```python
from build123d import *

# Parameters (mm, degrees)
SKETCH1_R           = 1.27
BOSS_EXTRUDE1_DEPTH = 2.5
FILLET1_R           = 5.08
CUT_EXTRUDE1_DEPTH  = 14.648809639
FILLET2_R           = 1.27


with BuildPart() as part:
    # Sketch1 → Boss-Extrude1 (new, symmetric)
    with BuildSketch(Plane(origin=(0, 0, 0), x_dir=(1, 0, 0), z_dir=(0, 1, 0))):
        with BuildLine():
            ThreePointArc((7.094482759, 2.780775861), (0, 7.62), (-7.094482759, 2.780775861))
            ThreePointArc((-7.094482759, 2.780775861), (-10.16, 0), (-7.094482759, -2.780775861))
            ThreePointArc((-7.094482759, -2.780775861), (0, -7.62), (7.094482759, -2.780775861))
            ThreePointArc((7.094482759, -2.780775861), (10.16, 0), (7.094482759, 2.780775861))
        make_face()
        with Locations(Location((7.366, 0, 0), (0, 0, 270))):
            Circle(SKETCH1_R, mode=Mode.SUBTRACT)
        with Locations(Location((-7.366, 0, 0), (0, 0, 270))):
            Circle(SKETCH1_R, mode=Mode.SUBTRACT)
    extrude(amount=BOSS_EXTRUDE1_DEPTH, both=True)

    # Fillet1
    fillet1_edges = [part.edges().sort_by_distance(p)[0] for p in [
        (-7.094482759, 0, 2.780775861),
        (-7.094482759, 0, -2.780775861),
        (7.094482759, 0, -2.780775861),
        (7.094482759, 0, 2.780775861),
    ]]
    fillet(fillet1_edges, radius=FILLET1_R)

    # Sketch2 → Cut-Extrude1 (cut, through all)
    with BuildSketch(Plane(origin=(0, 2.5, 0), x_dir=(1, 0, 0), z_dir=(0, 1, 0))):
        with BuildLine():
            ThreePointArc((5.213513626, 2.46164628), (4.096, 0), (5.213513626, -2.46164628))
            ThreePointArc((5.213513626, -2.46164628), (4.900166041, -2.826173582), (4.612275862, -3.21112307))
            ThreePointArc((4.612275862, -3.21112307), (0, -5.62), (-4.612275862, -3.21112307))
            ThreePointArc((-4.612275862, -3.21112307), (-4.900166041, -2.826173582), (-5.213513626, -2.46164628))
            ThreePointArc((-5.213513626, -2.46164628), (-4.096, 0), (-5.213513626, 2.46164628))
            ThreePointArc((-5.213513626, 2.46164628), (-4.900166041, 2.826173582), (-4.612275862, 3.21112307))
            ThreePointArc((-4.612275862, 3.21112307), (0, 5.62), (4.612275862, 3.21112307))
            ThreePointArc((4.612275862, 3.21112307), (4.900166041, 2.826173582), (5.213513626, 2.46164628))
        make_face()
    extrude(amount=-CUT_EXTRUDE1_DEPTH, mode=Mode.SUBTRACT)

    # Fillet2
    fillet2_edges = [part.edges().sort_by_distance(p)[0] for p in [
        (5.213513626, 0, -2.46164628),
        (-5.213513626, 0, -2.46164628),
        (-5.213513626, 0, 2.46164628),
        (5.213513626, 0, 2.46164628),
    ]]
    fillet(fillet2_edges, radius=FILLET2_R)


solid = part.part
```
The listing builds one solid part. Answer for the finished solid, in the listing's coordinates (mm). A direction names the side the tool comes from. Round coordinates to 2 decimals unless told otherwise and drop trailing zeros. Write each loop counter-clockwise with the first axis right and the second up, starting at its lowest first coordinate (ties: lowest second). Pieces come first, ordered by that corner, then holes. Notation, with made-up numbers: (-24, 14.25) -> (-18, 14.25) arc R18 ccw to (-18, 48.25) -> close; hole circle Ø6 at (-7.75, 85.25). An arc over 180 degrees is marked (long way). Answer as a JSON object with one key per item and string values. Group by question number.
Q1. Section D-D (z = -6) is taken. Write down the section's boundary in (x, y).
Q2. Which of the six approach directions +Z, -Z, +X, -X, +Y, -Y give full straight-line access (tool end or side, diameter ignored) to faces 1 (the face through (0.08, 0.03, 5.62)), 2 (the face through (-5, -2.5, 0))?
Q3. Straight lines are drawn through the part: line 1 along X through (y, z) = (1.35, 0); line 2 along X through (y, z) = (-1.9, -0.5); line 3 along Z through (x, y) = (-0.5, 1.25). For each, find the intervals that lie inside material, in ascending order.
Q4. Each of these flat-tipped pins is pushed along its axis until it touches: pin 1 Ø1 at (x, z) = (8, -6) entering from -Y; pin 2 Ø1 at (x, y) = (1.5, 2) entering from +Z; pin 3 Ø3.5 at (x, z) = (-7.366, 0) entering from +Y. Where does it stop, or does it pass through?
Q5. Determine the mould class of faces 3 (the face through (-4.096, 0.035, 0.027)), 4 (the face through (4.096, 0.035, -0.027)), 5 (the face through (-5, 2.5, 0)), 6 (the face through (0.1, 0.04, -7.62)) for opening direction X: pulls with the +X half, pulls with the -X half, needs draft (parallel to the pull), parting line crosses it, or undercut.
Q6. Section C-C (y = -2.2) is taken. Count the separate pieces of the cut face and the enclosed holes in it, plus the area to 3 significant figures.
Q7. Section A-A (z = 0) is taken. Write down the section's boundary in (x, y), plus the area to 3 significant figures.
Q8. Section B-B (x = -3) is taken. Write down the section's boundary in (y, z).
Check values:
{
 "1": {"outline": "(-4.7, -2.5) -> (4.7, -2.5) -> (4.7, 2.5) -> (-4.7, 2.5) -> close"},
 "2": {"face 1": "+Y, -Y", "face 2": "+Z, -Z, +X, -X, -Y"},
 "3": {"line 1": "-10.16 to -8.64, -6.1 to -4.1, 4.1 to 6.1, 8.64 to 10.16", "line 2": "-10.11 to -8.53, -6.2 to -4.13, 4.13 to 6.2, 8.53 to 10.11", "line 3": "-7.6 to -5.6, 5.6 to 7.6"},
 "4": {"pin 1": "through", "pin 2": "z = 7.55", "pin 3": "y = 2.5"},
 "5": {"face 3": "undercut", "face 4": "undercut", "face 5": "needs draft", "face 6": "parting line crosses it"},
 "6": {"separate pieces": "1", "enclosed holes": "3", "area": "109 mm^2"},
 "7": {"outline": "(-10.16, -2.5) -> (-8.64, -2.5) -> (-8.64, 2.5) -> (-10.16, 2.5) -> close; (-6.1, -2.5) -> (-4.1, -2.5) -> (-4.1, 2.5) -> (-6.1, 2.5) -> close; (4.1, -2.5) -> (6.1, -2.5) -> (6.1, 2.5) -> (4.1, 2.5) -> close; (8.64, -2.5) -> (10.16, -2.5) -> (10.16, 2.5) -> (8.64, 2.5) -> close", "area": "35.2 mm^2"},
 "8": {"outline": "(-2.5, -7) -> (2.5, -7) -> (2.5, -4.75) -> (-2.5, -4.75) -> close; (-2.5, 4.75) -> (2.5, 4.75) -> (2.5, 7) -> (-2.5, 7) -> close"}
}
